Geometry: see drawing. Coordinates: mm, zero at the bounding-box minimum. A direction names the side the tool comes from. Round coordinates to 2 decimals unless told otherwise and drop trailing zeros. Loops run counter-clockwise (first coordinate to the right, second up) from the corner with the lowest first, then second, coordinate; pieces in that order, holes last. Notation, with made-up numbers: (-20.5, 34.5) - (32.5, 34.5) arc R26 ccw to (32.5, 50.5) - close; hole circle Ø9 at (20, 59). An arc over 180 degrees is marked (long way). Return JSON: item names as keys, results as strings. Group by question number.
1. First-contact query: pin 1 Ø2 at (x, z) = (81.5, 67) entering from +Y. Flat tip, straight axial feed; report the tip coordinate or a pass-through.
2. Set-up query: the marked faces 5, 6 and 7. Return all of +Z, -Z, +X, -X, +Y, -Y with unobstructed straight access to the full face (end or side cutting, diameter ignored); none if empty.
3. Section B-B on x = 41.5. Return loops of the section in (y, z).
4. Material intervals for probe 1 along Y at (x, z) = (57.5, 66); probe 2 along Z at (x, y) = (28, 232.5), sorted ascending.
5. Draft query along Y for the marked faces 1, 2, 3 and 4. Return one class per face: +Y half, -Y half, draft (parallel to the pull), parting line (faces both ways), or undercut.
6. Section A-A on z = 69. Return loops of the section in (x, y).
7. Section C-C on y = 261.5. Return loops of the section in (x, z).
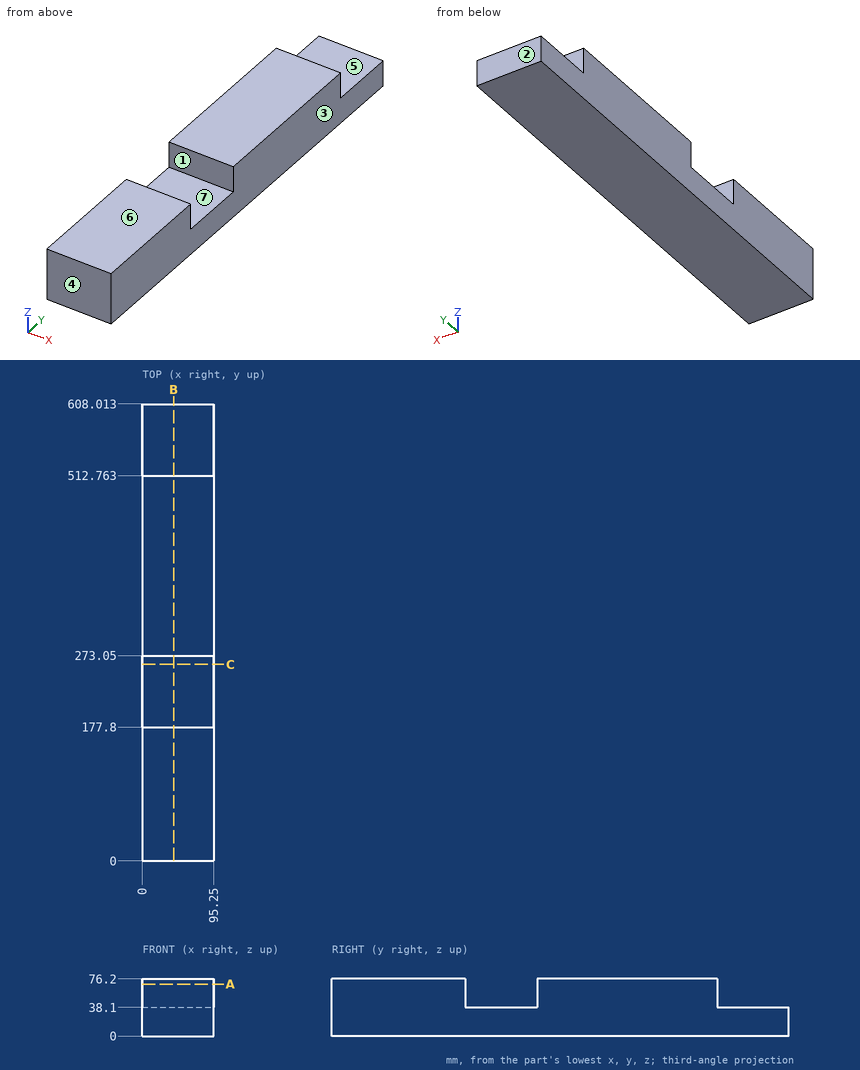
Taken from the geometry:
{
 "1": {"pin 1": "y = 512.76"},
 "2": {"face 5": "+Z, +X, -X, +Y", "face 6": "+Z, +X, -X, +Y, -Y", "face 7": "+Z, +X, -X"},
 "3": {"outline": "(0, 0) - (608.01, 0) - (608.01, 38.1) - (512.76, 38.1) - (512.76, 76.2) - (273.05, 76.2) - (273.05, 38.1) - (177.8, 38.1) - (177.8, 76.2) - (0, 76.2) - close"},
 "4": {"probe 1": "0 to 177.8, 273.05 to 512.76", "probe 2": "0 to 38.1"},
 "5": {"face 1": "undercut", "face 2": "+Y half", "face 3": "draft", "face 4": "-Y half"},
 "6": {"outline": "(0, 0) - (95.25, 0) - (95.25, 177.8) - (0, 177.8) - close; (0, 273.05) - (95.25, 273.05) - (95.25, 512.76) - (0, 512.76) - close"},
 "7": {"outline": "(0, 0) - (95.25, 0) - (95.25, 38.1) - (0, 38.1) - close"}
}
